Autodesk Inventor part; units mm, degrees
ref_plane "YZ Plane" through (0, 0, 0) normal (1, 0, 0) x (0, 1, 0)
ref_plane "XZ Plane" through (0, 0, 0) normal (0, 1, 0) x (-1, 0, 0)
ref_plane "XY Plane" through (0, 0, 0) normal (0, 0, 1) x (1, 0, 0)
sketch "Sketch1" plane through (0, 0, 0) normal (0, 0, 1) x (1, 0, 0)
  line L0 (-30.7315, 6.2426) -> (-15.7315, 6.2426)
  line L1 (-15.7315, 6.2426) -> (-15.7315, -8.7574)
  line L2 (-15.7315, -8.7574) -> (-30.7315, -8.7574)
  line L3 (-30.7315, -8.7574) -> (-30.7315, 6.2426)
  line L4 (0.2685, 2.2426) -> (0.2685, 12.2426)
  line L5 (0.2685, 12.2426) -> (-15.7315, 12.2426)
  line L6 (-15.7315, 12.2426) -> (-15.7315, 6.2426)
  line L7 (-15.7315, -8.7574) -> (0.2685, 2.2426)
  point P0 (0, 0)
  dimension "d0" = 15
  dimension "d1" = 15
  dimension "d2" = 6
  dimension "d3" = 16
  dimension "d4" = 10
extrude "Extrusion1" add sketch "Sketch1" along normal blind 16
sketch "Sketch2" plane through (-15.7315, 12.2426, 0) normal (0, 1, 0) x (1, 0, 0)
  line L0 (16, 0) -> (16, -16)
  line L1 (0, -5.3333) -> (16, -5.3333)
  line L2 (16, -5.3333) -> (16, -10.6667)
  line L3 (16, -10.6667) -> (0, -10.6667)
  line L4 (0, -10.6667) -> (0, -5.3333)
  line L5 (0, 0) -> (0, -16)
  line L6 (16, 0) -> (0, 0)
  line L7 (16, -16) -> (0, -16)
  point P0 (15.7315, 0)
  dimension "d7" = 16
  dimension "d8" = 5.3333
  dimension "d9" = 5.3333
extrude "Extrusion2" cut sketch "Sketch2" against normal blind 2 contours L0 L3 L4 L1
sketch "Sketch3" plane through (0.2685, 2.2426, 0) normal (1, 0, 0) x (0, 0, -1)
  line L0 (-10.6667, 8) -> (-10.6667, 10)
  line L1 (-10.6667, 10) -> (-16, 10)
  line L2 (-16, 0) -> (-16, 10)
  line L3 (0, 0) -> (-16, 0)
  line L4 (0, 0) -> (0, 10)
  line L5 (0, 10) -> (-5.3333, 10)
  line L6 (-5.3333, 10) -> (-5.3333, 8)
  line L7 (-5.3333, 8) -> (-10.6667, 8)
  line L8 (0, 0) -> (-16, 0)
  line L9 (-10.6667, 8) -> (-5.3333, 8)
  line L10 (-10.6667, 8) -> (-10.6667, -2)
  line L11 (-10.6667, -2) -> (-5.3333, -2)
  line L12 (-5.3333, -2) -> (-5.3333, 8)
  point P0 (0, -2.2426)
  dimension "d14" = 10
  dimension "d15" = 10
extrude "Extrusion3" cut sketch "Sketch3" against normal blind 2 contours L7 L12 L3 L10 | L3 L12 L11 L10
sketch "Sketch4" plane through (-15.7315, -8.7574, 0) normal (0.5665, -0.824, 0) x (0.824, 0.5665, 0)
  line L0 (16.9894, 10.6667) -> (19.4165, 10.6667)
  line L1 (19.4165, 10.6667) -> (19.4165, 16)
  line L2 (0, 16) -> (19.4165, 16)
  line L3 (0, 0) -> (0, 16)
  line L4 (0, 0) -> (19.4165, 0)
  line L5 (19.4165, 0) -> (19.4165, 5.3333)
  line L6 (19.4165, 5.3333) -> (16.9894, 5.3333)
  line L7 (16.9894, 5.3333) -> (16.9894, 10.6667)
  line L8 (16.9894, 10.6667) -> (19.4165, 10.6667)
  line L9 (16.9894, 10.6667) -> (0, 10.6667)
  line L10 (0, 10.6667) -> (0, 5.3333)
  line L11 (0, 5.3333) -> (16.9894, 5.3333)
  line L12 (16.9894, 5.3333) -> (16.9894, 10.6667)
  point P0 (17.9247, 0)
  dimension "d17" = 19.4165
extrude "Extrusion4" cut sketch "Sketch4" against normal blind 2 contours L7 L11 L3 L9
chamfer "Chamfer1" distance 2 angle 45 1 edges at (-16.8645, -7.1093, 8)
sketch "Sketch5" plane through (-30.7315, -8.7574, 0) normal (-1, 0, 0) x (0, 0, 1)
  line L0 (6, 13) -> (10, 13)
  line L1 (10, 13) -> (10, 2)
  line L2 (10, 2) -> (6, 2)
  line L3 (6, 2) -> (6, 13)
  line L4 (0, 15) -> (0, 0)
  line L5 (0, 0) -> (16, 0)
  line L6 (16, 15) -> (16, 0)
  line L7 (0, 15) -> (16, 15)
  point P0 (0, 8.7574)
  dimension "d23" = 4
  dimension "d24" = 11
  dimension "d25" = 6
  dimension "d26" = 15
  dimension "d27" = 16
  dimension "d28" = 2
extrude "Extrusion5" cut sketch "Sketch5" against normal blind 5 contours L0 L1 L2 L3
equation "\"d8\" = 0.333333 * d7"
equation "\"d9\" = -2 * d8 + d7"
equation "\"d14\" = d15"
equation "\"d25\" = -0.5 * d23 + 0.5 * d27"
equation "\"d28\" = -0.5 * d24 + 0.5 * d26"
properties part number "under walle L3"
The model under review builds one solid part; all positions refer to its coordinate system, in mm. A direction names the side the tool comes from. Coordinates: 2 decimals unless noted, no trailing zeros. Write each loop counter-clockwise with the first axis right and the second up, starting at its lowest first coordinate (ties: lowest second). Pieces come first, ordered by that corner, then holes.
1) The part is to be moulded in two halves that separate along Z. For faces 1 (the face through (-9, -3, 10.667)), 2 (the face through (0.268, 7, 3)), say which applies: pulls with the +Z half, pulls with the -Z half, needs draft (parallel to the pull), parting line crosses it, or undercut.
2) We need section D-D on x = -20. State the section outline as (y, z) points, then the cut area to 3 significant figures.
3) To check wall thickness, follow probe 1 along Z at (x, y) = (-27, -6.25); probe 2 along Z at (x, y) = (-5.5, 10.75); probe 3 along Y at (x, z) = (-22.5, 13.5). State the ranges of each line that lie inside material, in increasing order.
4) Machinability: for faces 3 (the face through (-15.732, 9, 8)), 4 (the face through (-9, 10.243, 8)), 5 (the face through (-9.13, -1.79, 8.04)), 6 (the face through (-28, -1, 10)), 7 (the face through (-4.7, 10.4, 10.667)), which of the approach directions +Z, -Z, +X, -X, +Y, -Y give a long, thin tool a straight path to every point of the face, cutting with its end or side? Answer none if there is none.
5) We need section A-A on y = 11.25. State the section outline as (x, z) points.
6) We need section C-C on y = 8.5. State the section outline as (x, z) points, then the cut area to 3 significant figures.
7) Clearance check with flat-ended pins moving along their axes: pin 1 Ø3 at (y, z) = (-6, 2.5) entering from +X; pin 2 Ø3 at (y, z) = (8, 11) entering from -X; pin 3 Ø1.5 at (y, z) = (-4.5, 8) entering from +X. State where each tip first meets the part, or that it passes through.
8) We need section B-B on z = 12.25. State the section outline as (x, y) points, then the cut area to 3 significant figures.
Answer list:
1. face 1: undercut
1. face 2: needs draft
2. outline: (-8.76, 0) - (6.24, 0) - (6.24, 16) - (-8.76, 16) - close
2. area: 240 mm2
3. probe 1: z = 0 to 6, 10 to 16
3. probe 2: z = 0 to 5.33, 10.67 to 16
3. probe 3: y = -8.76 to 6.24
4. face 3: +Z, -Z, -X, +Y
4. face 4: +X, -X, +Y
4. face 5: -Y
4. face 6: -X
4. face 7: +X, +Y
5. outline: (-15.73, 0) - (0.27, 0) - (0.27, 5.33) - (-15.73, 5.33) - close; (-15.73, 10.67) - (0.27, 10.67) - (0.27, 16) - (-15.73, 16) - close
6. outline: (-15.73, 0) - (0.27, 0) - (0.27, 5.33) - (-1.73, 5.33) - (-1.73, 10.67) - (0.27, 10.67) - (0.27, 16) - (-15.73, 16) - close
6. area: 245 mm2
7. pin 1: stops at x = -9.54
7. pin 2: stops at x = -15.73
7. pin 3: stops at x = -11.98
8. outline: (-30.73, -8.76) - (-15.73, -8.76) - (0.27, 2.24) - (0.27, 12.24) - (-15.73, 12.24) - (-15.73, 6.24) - (-30.73, 6.24) - close
8. area: 473 mm2
